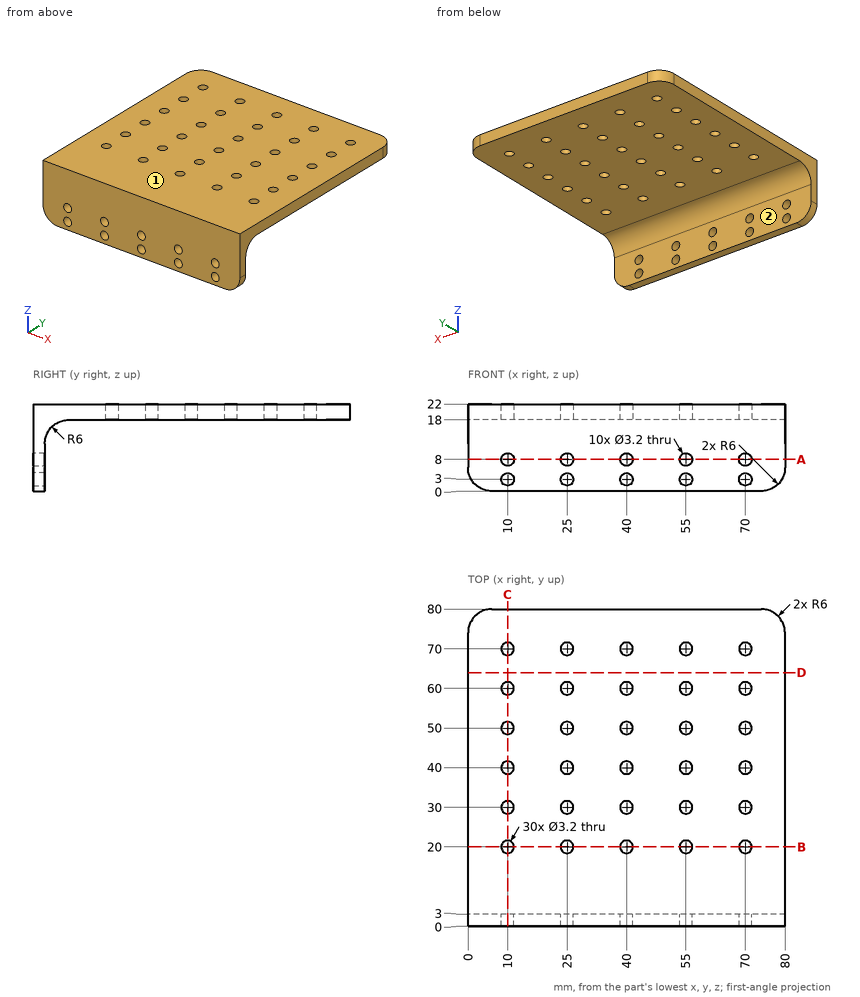
Verification items for this drawing (mm, ordinates from the low corner). A direction names the side the tool comes from. Coordinates: 2 decimals unless noted, no trailing zeros. Loops run counter-clockwise (first coordinate to the right, second up) from the corner with the lowest first, then second, coordinate; pieces in that order, holes last. Notation, with made-up numbers: (88.5, 30.5) - (102.5, 30.5) arc R11 ccw to (102.5, 43.5) - close; hole circle Ø1 at (83, 40). An arc over 180 degrees is marked (long way). Answer as a JSON object with one key per item and string values.
(1) Cross-section at B-B, the plane y = 20. Record the boundary of the cut face in (x, z), then the cut area to 3 significant figures.
Response:
{"outline": "(0, 18) - (8.4, 18) - (8.4, 22) - (0, 22) - close; (11.6, 18) - (23.4, 18) - (23.4, 22) - (11.6, 22) - close; (26.6, 18) - (38.4, 18) - (38.4, 22) - (26.6, 22) - close; (41.6, 18) - (53.4, 18) - (53.4, 22) - (41.6, 22) - close; (56.6, 18) - (68.4, 18) - (68.4, 22) - (56.6, 22) - close; (71.6, 18) - (80, 18) - (80, 22) - (71.6, 22) - close", "area": "256 mm²"}
(2) Cross-section at D-D, the plane y = 64. Record the boundary of the cut face in (x, z).
Response:
{"outline": "(0, 18) - (80, 18) - (80, 22) - (0, 22) - close"}
(3) Cross-section at C-C, the plane x = 10. Count the separate pieces of the cut face and the enclosed holes in it, then the cut area to 3 significant figures.
Response:
{"separate pieces": "9", "enclosed holes": "0", "area": "286 mm²"}
(4) Scan lines: line 1 along X through (y, z) = (70, 19.9); line 2 along Z through (x, y) = (50.5, 46); line 3 along Y through (x, z) = (59.5, 10.25). Record each from-to range of solid material in increasing order.
Response:
{"line 1": "x = 0 to 8.4, 11.6 to 23.4, 26.6 to 38.4, 41.6 to 53.4, 56.6 to 68.4, 71.6 to 80", "line 2": "z = 18 to 22", "line 3": "y = 0 to 3"}
(5) Cross-section at A-A, the plane z = 8. Record the boundary of the cut face in (x, y), then the cut area to 3 significant figures.
Response:
{"outline": "(0, 0) - (8.4, 0) - (8.4, 3) - (0, 3) - close; (11.6, 0) - (23.4, 0) - (23.4, 3) - (11.6, 3) - close; (26.6, 0) - (38.4, 0) - (38.4, 3) - (26.6, 3) - close; (41.6, 0) - (53.4, 0) - (53.4, 3) - (41.6, 3) - close; (56.6, 0) - (68.4, 0) - (68.4, 3) - (56.6, 3) - close; (71.6, 0) - (80, 0) - (80, 3) - (71.6, 3) - close", "area": "192 mm²"}
(6) Access from +Z, -Z, +X, -X, +Y, -Y to the whole of each face (thin tool, end or side, straight path). Record for the marked faces 1 and 2.
Response:
{"face 1": "+Z, +X, -X, +Y, -Y", "face 2": "-Z, +X, -X, +Y"}
(7) Go/stop test with flat-tipped pins: pin 1 Ø9.5 at (x, z) = (29, 8) entering from +Y; pin 2 Ø4 at (x, y) = (25, 20) entering from -Z; pin 3 Ø2 at (x, z) = (58, 15) entering from +Y. Record where each tip stops, or that it passes through.
Response:
{"pin 1": "stops at y = 3.05", "pin 2": "stops at z = 18", "pin 3": "stops at y = 4.53"}
